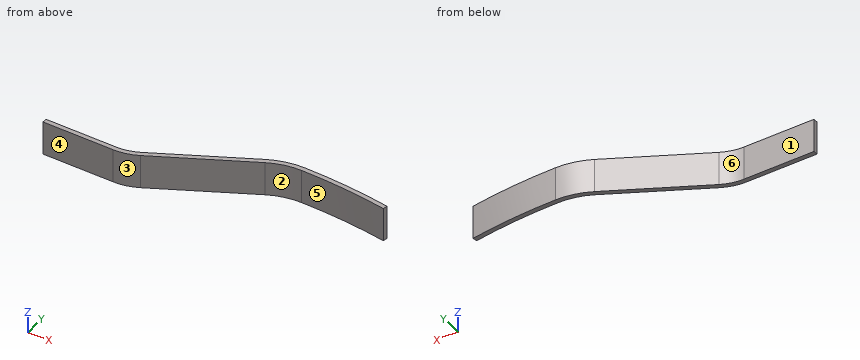
from build123d import *

# Parameters (mm, degrees)
F1_DEPTH = 15


with BuildPart() as f1:
    # F0 (on Top) → F1 (new body)
    with BuildSketch(Plane.XY):
        with BuildLine():
            Line((0, 2), (0, 0))
            Line((0, 0), (31.39012, 0))
            ThreePointArc((31.39012, 0), (36.833363, 0.668346), (41.95323, 2.633679))
            Line((41.95323, 2.633679), (83.010293, 24.464107))
            ThreePointArc((83.010293, 24.464107), (89.836783, 27.084551), (97.09444, 27.975679))
            ThreePointArc((97.09444, 27.975679), (116.452329, 27.225097), (135.693981, 24.977856))
            Line((135.693981, 24.977856), (136.002777, 26.953874))
            ThreePointArc((136.002777, 26.953874), (116.607192, 29.219092), (97.09444, 29.975679))
            ThreePointArc((97.09444, 29.975679), (89.352939, 29.025142), (82.07135, 26.230002))
            Line((82.07135, 26.230002), (41.014287, 4.399574))
            ThreePointArc((41.014287, 4.399574), (36.349519, 2.608938), (31.39012, 2))
            Line((31.39012, 2), (0, 2))
        make_face()
    extrude(amount=F1_DEPTH)


solid = f1.part
Check sheet for the modelled part. Datum: model origin and axes. Units: mm. Face numbers are marked on the shaded views. A direction names the side the tool comes from. Coordinates: 2 decimals unless noted, no trailing zeros. Write each loop counter-clockwise with the first axis right and the second up, starting at its lowest first coordinate (ties: lowest second). Pieces come first, ordered by that corner, then holes.
Item 1: Mould release check, pull along X, two halves, no side actions. Record for the marked faces 4, 5 and 6: released by +X, released by -X, zero draft, split by the parting line, or undercut.
Numbers:
face 4: zero draft
face 5: undercut
face 6: released by -X
Item 2: Cross-section at B-B on x = 76. Record the boundary of the cut face in (y, z), then the cut area to 3 significant figures.
Numbers:
outline: (20.74, 0) - (23, 0) - (23, 15) - (20.74, 15) - close
area: 34.0 mm2
Item 3: Depth check by flat-ended pin: pin 1 Ø1.5 at (y, z) = (3, 11) entering from +X; pin 2 Ø8 at (y, z) = (11.5, 6.5) entering from +X; pin 3 Ø8 at (x, y) = (111.5, 25.5) entering from +Z; pin 4 Ø1.5 at (y, z) = (18.5, 11.5) entering from -X. Enter the tip coordinate at first touch or a pass-through.
Numbers:
pin 1: stops at x = 44.05
pin 2: stops at x = 66.15
pin 3: stops at z = 15
pin 4: stops at x = 66.12
Item 4: Scan lines: probe 1 along Y at (x, z) = (23, 1.75); probe 2 along Y at (x, z) = (67.5, 4.5); probe 3 along X at (y, z) = (8.5, 9.5). Record each from-to range of solid material in increasing order.
Numbers:
probe 1: y = 0 to 2
probe 2: y = 16.22 to 18.48
probe 3: x = 48.73 to 52.99
Item 5: Access from +Z, -Z, +X, -X, +Y, -Y to the whole of each face (thin tool, end or side, straight path). Record for the marked faces 1, 2 and 3.
Numbers:
face 1: +Z, -Z, -X, +Y
face 2: +Z, -Z, -Y
face 3: +Z, -Z, +X, -Y
Item 6: Cross-section at A-A on z = 3.25. Record the boundary of the cut face in (x, y).
Numbers:
outline: (0, 0) - (31.39, 0) arc R22.5 ccw to (41.95, 2.63) - (83.01, 24.46) arc R30 cw to (97.09, 27.98) arc R250 cw to (135.69, 24.98) - (136, 26.95) arc R252 ccw to (97.09, 29.98) arc R32 ccw to (82.07, 26.23) - (41.01, 4.4) arc R20.5 cw to (31.39, 2) - (0, 2) - close
Item 7: Cross-section at C-C on y = 15. Record the boundary of the cut face in (x, z).
Numbers:
outline: (60.95, 0) - (65.21, 0) - (65.21, 15) - (60.95, 15) - close
